Input: part model. Units: mm. Frame: model coordinates. Face numbers are marked on the shaded views. A direction names the side the tool comes from. Give positions to 0.01 mm unless a question says otherwise; leave off trailing zeros. Write each loop counter-clockwise with the first axis right and the second up, starting at its lowest first coordinate (ties: lowest second). Pieces come first, ordered by that corner, then holes.
```python
from build123d import *

# Parameters (mm, degrees)
SKETCH1_W           = 50
SKETCH1_H           = 35
BOSS_EXTRUDE1_DEPTH = 3.5
SKETCH2_R           = 1.85
CUT_EXTRUDE1_DEPTH  = 31.716445107
SKETCH3_R           = 3.5
BOSS_EXTRUDE2_DEPTH = 25
CUT_EXTRUDE2_START  = 8.2
CUT_EXTRUDE2_DEPTH  = 8.2


with BuildPart() as part:
    # Sketch1 → Boss-Extrude1 (new body)
    with BuildSketch(Plane(origin=(0, 0, 0), x_dir=(1, 0, 0), z_dir=(0, 1, 0))):
        Rectangle(SKETCH1_W, SKETCH1_H)
    extrude(amount=BOSS_EXTRUDE1_DEPTH)

    # Sketch2 → Cut-Extrude1 (cut, through all)
    with BuildSketch(Plane(origin=(0, 3.5, 0), x_dir=(1, 0, 0), z_dir=(0, 1, 0))):
        with Locations(Location((0, -8, 0), (0, 0, 270))):
            Circle(SKETCH2_R)
        with Locations(Location((16.6, 2.45, 0), (0, 0, 270))):
            Circle(SKETCH2_R)
        with Locations(Location((-16.6, 2.45, 0), (0, 0, 270))):
            Circle(SKETCH2_R)
    extrude(amount=-CUT_EXTRUDE1_DEPTH, mode=Mode.SUBTRACT)

    # Sketch3 → Boss-Extrude2 (add, symmetric)
    with BuildSketch(Plane(origin=(0, 0, 0), x_dir=(0, 0, -1), z_dir=(1, 0, 0))):
        with BuildLine():
            Line((17.5, 0), (19.401351351, -2.633887439))
            ThreePointArc((19.401351351, -2.633887439), (27.235272499, -1.653328191), (22.186446019, 4.416364401))
            Line((22.186446019, 4.416364401), (17.5, 3.5))
            Line((17.5, 3.5), (17.5, 1.655278421))
            Line((17.5, 1.655278421), (17.5, 0))
        make_face()
        with Locations((23.05, 0)):
            Circle(SKETCH3_R, mode=Mode.SUBTRACT)
    extrude(amount=BOSS_EXTRUDE2_DEPTH, both=True)

    # Sketch4 → Cut-Extrude2 (cut)
    with BuildSketch(Plane(origin=(7.9, 0, 0), x_dir=(0, 0, -1), z_dir=(1, 0, 0)).offset(CUT_EXTRUDE2_START)):
        with BuildLine():
            Line((17.5, 3.5), (17.5, 0))
            Line((17.5, 0), (19.401351351, -2.633887439))
            ThreePointArc((19.401351351, -2.633887439), (27.235272499, -1.653328191), (22.186446019, 4.416364401))
            Line((22.186446019, 4.416364401), (17.5, 3.5))
        make_face()
    cut_extrude2 = extrude(amount=-CUT_EXTRUDE2_DEPTH, mode=Mode.SUBTRACT)

    # Mirror1: Cut-Extrude2 across plane
    add(cut_extrude2.mirror(Plane(origin=(0, 0, 0), x_dir=(0, 0, 1), z_dir=(1, 0, 0))), mode=Mode.SUBTRACT)


solid = part.part
```
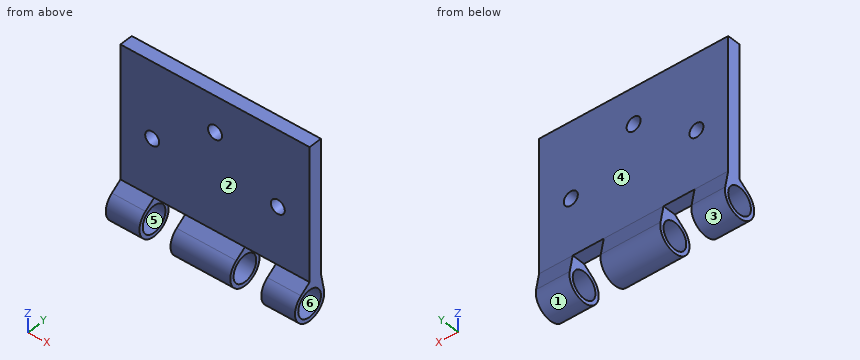
Item 1: Section D-D (z = -2.45). Return loops of the section in (x, y).
Item 2: Pin query (flat end, axial travel): pin 1 (17.5 mm diameter, centred on x = -10.5, z = -5, fed in from -Y); pin 2 (3 mm diameter, centred on x = 13, y = 2.5, fed in from -Z); pin 3 (2 mm diameter, centred on x = 4.5, y = -2, fed in from +Z). Return the tip coordinate at first contact, or that it passes through.
Item 3: Mould query, pull axis Z, two halves, no side actions, for the marked faces 3, 4, 5 and 6. Classes: +Z half, -Z half, draft (parallel to the pull), parting line (faces both ways), or undercut.
Item 4: Section A-A (x = 0). Return loops of the section in (y, z), and give its area (3 significant figures).
Item 5: Ray query, line 1 (X direction, y = 2.75, z = -2.45); line 2 (X direction, y = -1.25, z = -18.5); line 3 (Z direction, x = -18, y = 1.5). Return the intervals inside material, ascending.
Item 6: Section B-B (z = 8). Return loops of the section in (x, y).
Item 7: Section C-C (y = 2.75). Return loops of the section in (x, z), and give its area (3 significant figures).
Item 8: Set-up query: the marked faces 1 and 2. Return all of +Z, -Z, +X, -X, +Y, -Y with unobstructed straight access to the full face (end or side cutting, diameter ignored); none if empty.
Solved:
1. outline: (-25, 0) - (-18.45, 0) - (-18.45, 3.5) - (-25, 3.5) - close; (-14.75, 0) - (14.75, 0) - (14.75, 3.5) - (-14.75, 3.5) - close; (18.45, 0) - (25, 0) - (25, 3.5) - (18.45, 3.5) - close
2. pin 1: stops at y = 0
2. pin 2: stops at z = -17.5
2. pin 3: stops at z = -18.22
3. face 3: parting line
3. face 4: draft
3. face 5: undercut
3. face 6: undercut
4. outline: (-2.63, -19.4) arc R4.5 ccw (long way) to (4.42, -22.19) - (3.5, -17.5) - (3.5, 6.15) - (0, 6.15) - (0, -17.5) - close; (0, 9.85) - (3.5, 9.85) - (3.5, 17.5) - (0, 17.5) - close; hole circle Ø7 at (0, -23.05)
4. area: 142 mm2
5. line 1: x = -25 to -18.45, -14.75 to 14.75, 18.45 to 25
5. line 2: x = -25 to -16.1, -7.9 to 7.9, 16.1 to 25
5. line 3: z = -27.29 to -26.21, -19.89 to -3.66, -1.24 to 17.5
6. outline: (-25, 0) - (-1.85, 0) - (-1.85, 3.5) - (-25, 3.5) - close; (1.85, 0) - (25, 0) - (25, 3.5) - (1.85, 3.5) - close
7. outline: (-25, -26.61) - (-16.1, -26.61) - (-16.1, -25.22) - (-25, -25.22) - close; (-25, -20.88) - (-16.1, -20.88) - (-16.1, -17.5) - (-7.9, -17.5) - (-7.9, -20.88) - (7.9, -20.88) - (7.9, -17.5) - (16.1, -17.5) - (16.1, -20.88) - (25, -20.88) - (25, 17.5) - (-25, 17.5) - close; (-7.9, -26.61) - (7.9, -26.61) - (7.9, -25.22) - (-7.9, -25.22) - close; (16.1, -26.61) - (25, -26.61) - (25, -25.22) - (16.1, -25.22) - close; hole circle Ø3.7 at (-16.6, -2.45); hole circle Ø3.7 at (0, 8); hole circle Ø3.7 at (16.6, -2.45)
7. area: 1,880 mm2
8. face 1: +X, -X
8. face 2: +Z, +X, -X, -Y
